```python
from build123d import *

# Parameters (mm, degrees)
SKETCH1_R           = 5.5
SKETCH1_R_2         = 1.5
BOSS_EXTRUDE1_DEPTH = 10
SKETCH2_W           = 9.9
SKETCH2_H           = 3
CUT_EXTRUDE1_DEPTH  = 2
SKETCH3_W           = 20.106266241
SKETCH3_H           = 11
CUT_EXTRUDE2_DEPTH  = 10
SKETCH4_R           = 1.5
CUT_EXTRUDE3_DEPTH  = 10
CUT_EXTRUDE4_DEPTH  = 3


with BuildPart() as part:
    # Sketch1 → Boss-Extrude1 (new body)
    with BuildSketch(Plane(origin=(0, 0, 0), x_dir=(1, 0, 0), z_dir=(0, 1, 0))):
        with BuildLine():
            Line((0, 0), (0, -75))
            Line((0, -75), (9.9, -75))
            Line((9.9, -75), (9.9, 0))
            Line((9.9, 0), (24.95, 0))
            Line((24.95, 0), (24.95, 4))
            ThreePointArc((24.95, 4), (35.95, 15), (24.95, 26))
            Line((24.95, 26), (0, 26))
            Line((0, 26), (0, 0))
        make_face()
        with Locations(Location((24.95, 15, 0), (0, 0, 270))):
            Circle(SKETCH1_R, mode=Mode.SUBTRACT)
        with Locations(Location((24.95, 23, 0), (0, 0, 270))):
            Circle(SKETCH1_R_2, mode=Mode.SUBTRACT)
        with Locations(Location((24.95, 7, 0), (0, 0, 270))):
            Circle(SKETCH1_R_2, mode=Mode.SUBTRACT)
        with Locations(Location((16.95, 15, 0), (0, 0, 270))):
            Circle(SKETCH1_R_2, mode=Mode.SUBTRACT)
    extrude(amount=BOSS_EXTRUDE1_DEPTH)

    # Sketch2 → Cut-Extrude1 (cut)
    with BuildSketch(Plane(origin=(0, 10, 0), x_dir=(1, 0, 0), z_dir=(0, 1, 0))):
        with Locations((4.95, -70.5)):
            Rectangle(SKETCH2_W, SKETCH2_H)
    extrude(amount=-CUT_EXTRUDE1_DEPTH, mode=Mode.SUBTRACT)

    # Sketch3 → Cut-Extrude2 (cut)
    with BuildSketch(Plane(origin=(0, 10, 0), x_dir=(1, 0, 0), z_dir=(0, 1, 0))):
        with Locations((35.003133121, 15)):
            Rectangle(SKETCH3_W, SKETCH3_H)
    extrude(amount=-CUT_EXTRUDE2_DEPTH, mode=Mode.SUBTRACT)

    # Sketch4 → Cut-Extrude3 (cut)
    with BuildSketch(Plane(origin=(0, 10, 0), x_dir=(1, 0, 0), z_dir=(0, 1, 0))):
        with Locations(Location((4.95, -10, 0), (0, 0, 270))):
            Circle(SKETCH4_R)
    extrude(amount=-CUT_EXTRUDE3_DEPTH, mode=Mode.SUBTRACT)

    # Sketch5 → Cut-Extrude4 (cut)
    with BuildSketch(Plane(origin=(0, 10, 0), x_dir=(1, 0, 0), z_dir=(0, 1, 0))):
        Polygon((4.95, -5), (0.619872981, -7.5), (0.619872981, -12.5), (4.95, -15), (9.280127019, -12.5), (9.280127019, -7.5), align=None)
    extrude(amount=-CUT_EXTRUDE4_DEPTH, mode=Mode.SUBTRACT)


solid = part.part
```
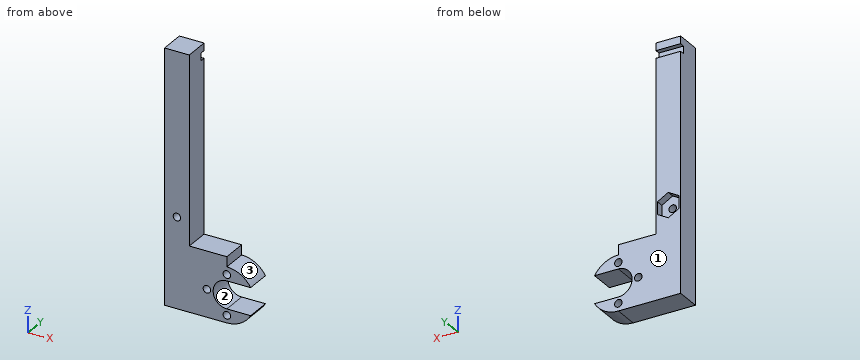
Model file for the job. Use its own axes, mm. Face numbers are marked on the shaded views. Coordinates: 2 decimals unless noted, no trailing zeros. Order: outer loops, then holes, each group sorted by start corner. A loop starts at its lowest first (then second) coordinate and runs counter-clockwise, first axis right, second up. Notation, with made-up numbers: (-32.5, 59.5) - (-3.5, 59.5) arc R34 cw to (-3.5, 92.5) - close; hole circle Ø10 at (38.5, -11.5). An arc over 180 degrees is marked (long way). Return JSON: item names as keys, results as strings. Group by question number.
1) Probe line 1 (X direction, y = 6.75, z = -15); line 2 (Z direction, x = 5, y = 8.25); line 3 (X direction, y = 1, z = 48.5). List the from-to ranges inside material, lowest first. Write a range as from..to.
2) Flat gauge pins, fed straight in: P1, Ø3.5, axis at y = 9, z = 9.5, coming from the +X side; P2, Ø8, axis at x = 12.5, z = 46, coming from the -Y side; P3, Ø4, axis at x = 17.5, y = 1.5, coming from the +Z side; P4, Ø2, axis at y = 5.5, z = -1.5, coming from the +X side. Where does each tip first touch, or does it go through?
3) Saw through at A-A, the plane z = -15. Write the cut outline in (x, y).
4) Saw through at D-D, the plane z = 41. Write the cut outline in (x, y), plus the area to 3 significant figures.
5) Saw through at B-B, the plane y = 3.75. Write the cut outline in (x, z), plus the area to 3 significant figures.
6) Saw through at C-C, the plane x = 32. Write the cut outline in (y, z), plus the area to 3 significant figures.
7) Mould opens along Z. For the marked faces 1, 2 and 3 say: released by +Z, released by -Z, zero draft, split by the parting line, or undercut.
Values found:
{
 "1": {"line 1": "x = 0..15.45, 18.45..19.45", "line 2": "z = -26..5.03, 14.97..69, 72..75", "line 3": "x = 0..9.9"},
 "2": {"P1": "stops at x = 9.9", "P2": "stops at y = 0", "P3": "stops at z = 0", "P4": "stops at x = 24.95"},
 "3": {"outline": "(0, 0) - (15.45, 0) - (15.45, 10) - (0, 10) - close; (18.45, 0) - (19.45, 0) - (19.45, 10) - (18.45, 10) - close"},
 "4": {"outline": "(0, 0) - (9.9, 0) - (9.9, 10) - (0, 10) - close", "area": "99.0 mm²"},
 "5": {"outline": "(0, -26) - (24.95, -26) arc R11 ccw to (34.48, -20.5) - (24.95, -20.5) arc R5.5 cw to (24.95, -9.5) - (34.48, -9.5) arc R11 ccw to (24.95, -4) - (24.95, 0) - (9.9, 0) - (9.9, 75) - (0, 75) - close; hole circle Ø3 at (4.95, 10); hole circle Ø3 at (16.95, -15); hole circle Ø3 at (24.95, -23); hole circle Ø3 at (24.95, -7)", "area": "1,390 mm²"},
 "6": {"outline": "(0, -23.44) - (10, -23.44) - (10, -20.5) - (0, -20.5) - close; (0, -9.5) - (10, -9.5) - (10, -6.56) - (0, -6.56) - close", "area": "58.9 mm²"},
 "7": {"face 1": "zero draft", "face 2": "undercut", "face 3": "released by +Z"}
}
